Can you work these out from the model? Positions are in its coordinate system, mm. Give positions to 0.01 mm unless a question says otherwise; leave off trailing zeros. Loops run counter-clockwise (first coordinate to the right, second up) from the corner with the lowest first, then second, coordinate; pieces in that order, holes last. Notation, with made-up numbers: (-24, 70.25) - (30, 70.25) arc R30 cw to (30, 102.25) - close; hole circle Ø10 at (60, 63.5). An arc over 180 degrees is marked (long way). Use a Markdown table: item, result. Add a question column.
```python
from build123d import *

# Parameters (mm, degrees)
F0_W     = 5
F0_H     = 5
F1_DEPTH = 5
F2_R     = 1.5
F3_DEPTH = 8.0264
F5_R     = 1.344016
F6_DEPTH = 20


with BuildPart() as f1:
    # F0 (on Top) → F1 (new body)
    with BuildSketch(Plane.XY):
        Rectangle(F0_W, F0_H)
    extrude(amount=F1_DEPTH)

    # F2 (on face) → F3 (cut)
    with BuildSketch(Plane.XY.offset(5)):
        Circle(F2_R)
    extrude(amount=-F3_DEPTH, mode=Mode.SUBTRACT)

    # F5 (on face) → F6 (cut)
    with BuildSketch(Plane.XZ.offset(2.5)):
        with Locations((0, 2.635571)):
            Circle(F5_R)
    extrude(amount=-F6_DEPTH, mode=Mode.SUBTRACT)


solid = f1.part
```
1. Suppose I cut it at B-B (y = -1.35). List the corners of the cut face in (x, z) for me.
2. Suppose I cut it at D-D (z = 4.55). List the corners of the cut face in (x, y) for me, and give its area (3 significant figures).
3. Suppose I cut it at C-C (z = 2.05). List the corners of the cut face in (x, y) for me.
4. If we mould it in two halves opening along X, with no side actions, what happens to faces 1 (the face through (2.5, 0, 2)), 2 (the face through (1.43, 0.45, 2.54)), 3 (the face through (0, 2, 0))? For each: released by +X, released by -X, zero draft, split by the parting line, or undercut.
5. Please list where these lines run through material, in increasing order: line 1 along Z through (x, y) = (0, -1.55); line 2 along X through (y, z) = (-1.3, 4.55); line 3 along X through (y, z) = (0.8, 0.6). Write a range as [from, to].
6. Suppose I cut it at A-A (x = 0). List the corners of the cut face in (y, z) for me.
Results below:
| question | item | result |
|---|---|---|
| 1 | outline | (-2.5, 0) - (-0.65, 0) - (-0.65, 1.46) arc R1.34 cw to (-0.65, 3.81) - (-0.65, 5) - (-2.5, 5) - close; (0.65, 0) - (2.5, 0) - (2.5, 5) - (0.65, 5) - (0.65, 3.81) arc R1.34 cw to (0.65, 1.46) - close |
| 2 | outline | (-2.5, -2.5) - (2.5, -2.5) - (2.5, 2.5) - (-2.5, 2.5) - close; hole circle Ø3 at (0, 0) |
| 2 | area | 17.9 mm² |
| 3 | outline | (-2.5, -2.5) - (-1.21, -2.5) - (-1.21, -0.89) arc R1.5 cw to (-1.21, 0.89) - (-1.21, 2.5) - (-2.5, 2.5) - close; (1.21, -2.5) - (2.5, -2.5) - (2.5, 2.5) - (1.21, 2.5) - (1.21, 0.89) arc R1.5 cw to (1.21, -0.89) - close |
| 4 | face 1 | released by +X |
| 4 | face 2 | undercut |
| 4 | face 3 | zero draft |
| 5 | line 1 | [0, 1.29], [3.98, 5] |
| 5 | line 2 | [-2.5, -0.75], [0.75, 2.5] |
| 5 | line 3 | [-2.5, -1.27], [1.27, 2.5] |
| 6 | outline | (-2.5, 0) - (-1.5, 0) - (-1.5, 1.29) - (-2.5, 1.29) - close; (-2.5, 3.98) - (-1.5, 3.98) - (-1.5, 5) - (-2.5, 5) - close; (1.5, 0) - (2.5, 0) - (2.5, 1.29) - (1.5, 1.29) - close; (1.5, 3.98) - (2.5, 3.98) - (2.5, 5) - (1.5, 5) - close |
